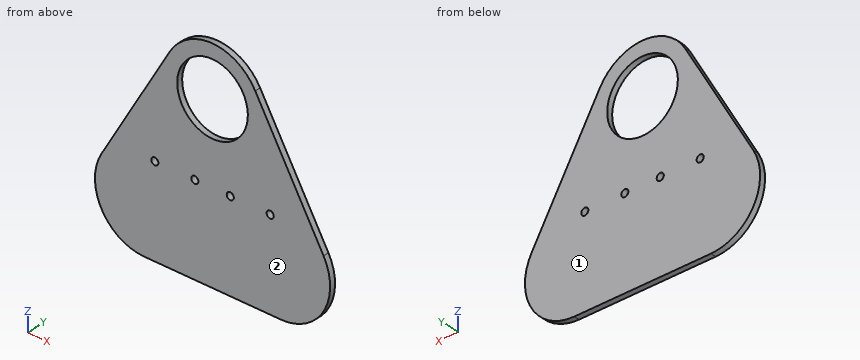
from build123d import *

# Parameters (mm, degrees)
BOSS_EXTRUDE1_DEPTH = 3.175
FILLET1_R           = 27.78
SKETCH5_R           = 2
CUT_EXTRUDE2_DEPTH  = 95.405671522
SKETCH7_R           = 1.5
SKETCH7_R_2         = 3.925
CUT_EXTRUDE3_DEPTH  = 10
SKETCH2_R           = 19.9
CUT_EXTRUDE4_DEPTH  = 95.405671522


with BuildPart() as part:
    # Sketch1 → Boss-Extrude1 (new body)
    with BuildSketch(Plane(origin=(0, 0, 0), x_dir=(1, 0, 0), z_dir=(0, 1, 0))):
        Polygon((0, -94.945058207), (-86.602540378, 55.054941793), (86.602540378, 55.054941793), align=None)
    extrude(amount=BOSS_EXTRUDE1_DEPTH)

    # Fillet1
    fillet1_edges = [part.edges().sort_by_distance(p)[0] for p in [
        (0, 1.5875, 94.945058207),
        (-86.602540378, 1.5875, -55.054941793),
        (86.602540378, 1.5875, -55.054941793),
    ]]
    fillet(fillet1_edges, radius=FILLET1_R)

    # Sketch5 → Cut-Extrude2 (cut, through all)
    with BuildSketch(Plane(origin=(0, 3.175, 0), x_dir=(1, 0, 0), z_dir=(0, 1, 0))):
        with Locations(Location((32.5, 5.054941793, 0), (0, 0, 270))):
            Circle(SKETCH5_R)
        with Locations(Location((-32.5, 5.054941793, 0), (0, 0, 270))):
            Circle(SKETCH5_R)
        with Locations(Location((-10, 5.054941793, 0), (0, 0, 270))):
            Circle(SKETCH5_R)
        with Locations(Location((10, 5.054941793, 0), (0, 0, 270))):
            Circle(SKETCH5_R)
    extrude(amount=-CUT_EXTRUDE2_DEPTH, mode=Mode.SUBTRACT)

    # Sketch7 → Cut-Extrude3 (cut)
    with BuildSketch(Plane(origin=(0, 3.175, 0), x_dir=(1, 0, 0), z_dir=(0, 1, 0))):
        with Locations(Location((0, -30.885058207, 0), (0, 0, 270))):
            Circle(SKETCH7_R)
        with Locations(Location((-7.361215932, -43.635058207, 0), (0, 0, 270))):
            Circle(SKETCH7_R)
        with Locations(Location((0, -39.385058207, 0), (0, 0, 270))):
            Circle(SKETCH7_R_2)
        with Locations(Location((7.361215932, -43.635058207, 0), (0, 0, 270))):
            Circle(SKETCH7_R)
    extrude(amount=-CUT_EXTRUDE3_DEPTH, mode=Mode.SUBTRACT)

    # Sketch2 → Cut-Extrude4 (cut, through all)
    with BuildSketch(Plane(origin=(0, 3.175, 0), x_dir=(1, 0, 0), z_dir=(0, 1, 0))):
        with Locations(Location((0, -39.385058207, 0), (0, 0, 270))):
            Circle(SKETCH2_R)
    extrude(amount=-CUT_EXTRUDE4_DEPTH, mode=Mode.SUBTRACT)


solid = part.part
Model file for the job. Use its own axes, mm. Face numbers are marked on the shaded views. Round coordinates to 2 decimals unless told otherwise and drop trailing zeros. Loops run counter-clockwise (first coordinate to the right, second up) from the corner with the lowest first, then second, coordinate; pieces in that order, holes last.
1. Band-saw the part on C-C, the plane z = 35.5. List the corners of the cut face in (x, y) (3 decimals), and give its area (3 significant figures).
Check values:
outline: (-34.321, 0) - (-19.517, 0) - (-19.517, 3.175) - (-34.321, 3.175) - close; (19.517, 0) - (34.321, 0) - (34.321, 3.175) - (19.517, 3.175) - close
area: 94.0 mm2
2. Mould opens along Y. For the marked faces 1 and 2 say: +Y half, -Y half, draft (parallel to the pull), parting line (faces both ways), or undercut.
Check values:
face 1: +Y half
face 2: -Y half
3. Band-saw the part on A-A, the plane x = 0. List the corners of the cut face in (y, z) (3 decimals).
Check values:
outline: (0, -55.055) - (3.175, -55.055) - (3.175, 19.485) - (0, 19.485) - close; (0, 59.285) - (3.175, 59.285) - (3.175, 67.165) - (0, 67.165) - close
4. Drop flat-ended pins along their axis: P1, Ø1.5, axis at y = 1, z = 21, coming from the -X side; P2, Ø1, axis at x = 49.5, y = 2, coming from the +Z side; P3, Ø2.5, axis at x = 10, z = -5.05, coming from the +Y side; P4, Ø1, axis at y = 1, z = -18, coming from the +X side. Give the stop position or say it passes through.
Check values:
P1: stops at x = -43.13
P2: stops at z = 10.07
P3: passes through
P4: stops at x = 64.84
5. Band-saw the part on B-B, the plane y = 2.3. List the corners of the cut face in (x, z), and give its area (3 significant figures).
Check values:
outline: (-62.54, -13.38) arc R27.78 ccw to (-38.49, -55.05) - (38.49, -55.05) arc R27.78 ccw to (62.54, -13.38) - (24.06, 53.28) arc R27.78 ccw to (-24.06, 53.28) - close; hole circle Ø4 at (-32.5, -5.05); hole circle Ø39.8 at (0, 39.39); hole circle Ø4 at (-10, -5.05); hole circle Ø4 at (10, -5.05); hole circle Ø4 at (32.5, -5.05)
area: 10,100 mm2
6. Band-saw the part on D-D, the plane z = 9. List the corners of the cut face in (x, y) (3 decimals).
Check values:
outline: (-49.62, 0) - (49.62, 0) - (49.62, 3.175) - (-49.62, 3.175) - close
7. Wall check: probe 1 along Z at (x, y) = (-1, 0.25); probe 2 along X at (y, z) = (2.7, -27); probe 3 along Z at (x, y) = (-31, 0.25). Give the ranges that are in metal, low to high.
Check values:
probe 1: z = -55.05 to 19.51, 59.26 to 67.15
probe 2: x = -66.26 to 66.26
probe 3: z = -55.05 to -6.38, -3.73 to 41.25
